Answer from the drawing. Dimensions are ordinates in mm from the lowest x, y and z of the part. A direction names the side the tool comes from. Give positions to 0.01 mm unless a question says otherwise; leave off trailing zeros. Put each result on its own line as item: value. Start each with the question number.
1. Given pin 1 Ø2 at (x, z) = (14.27, 4.75) entering from +Y; pin 2 Ø3 at (x, z) = (5.5, 4.5) entering from +Y (1 decimal), each flat-ended and moving along its own axis, determine where each tip first touches the part or whether it passes through.
2. For a pull along X with two mould halves and no side action, classify the marked faces 1, 2 and 3 as released by +X, released by -X, zero draft, split by the parting line, or undercut.
3. For the marked faces 4 and 5, determine the directions among +Z, -Z, +X, -X, +Y, -Y from which every point of the face is accessible in a straight line to the end or side of a thin tool.
4. A cutting plane is placed at B-B, the plane z = 6. Count the separate pieces of the cut face and the enclosed holes in it.
5. Consider L1, parallel to X at y = 4.5, z = 2.5; L2, parallel to Y at x = 4, z = 2.75 (1 decimal); L3, parallel to Z at x = 5.25, y = 1 (1 decimal). Determine where each line is inside the solid, lowest interval first. Write a range as from..to.
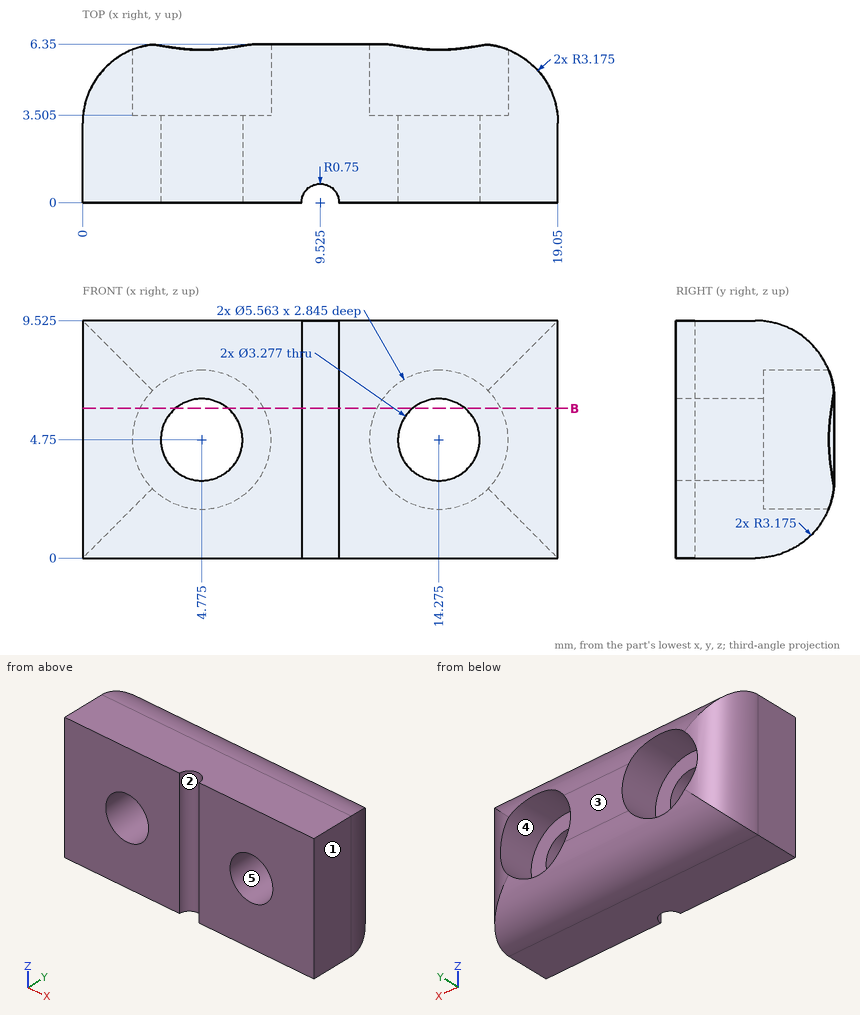
Return value:
1. pin 1: passes through
1. pin 2: stops at y = 3.5
2. face 1: released by +X
2. face 2: undercut
2. face 3: zero draft
3. face 4: +Y
3. face 5: +Y, -Y
4. separate pieces: 3
4. enclosed holes: 0
5. L1: x = 0.29..3.14, 6.41..12.64, 15.91..18.76
5. L2: y = 0..3.5
5. L3: z = 0..3.2, 6.3..9.5
